Check sheet for the modelled part. Datum: model origin and axes. Units: mm. A direction names the side the tool comes from. Round coordinates to 2 decimals unless told otherwise and drop trailing zeros. Loops run counter-clockwise (first coordinate to the right, second up) from the corner with the lowest first, then second, coordinate; pieces in that order, holes last. Notation, with made-up numbers: (49, -22.75) - (59, -22.75) arc R20 cw to (59, -8.75) - close; hole circle Ø6 at (18.5, -16). An arc over 180 degrees is marked (long way). Answer in a Markdown table with one row per item. Add a question column.
(1) Cross-section at C-C on z = 12. Count the separate pieces of the cut face and the enclosed holes in it, then the cut area to 3 significant figures.
(2) Gauge pin test, flat ends, axial feed: pin 1 (12.5 mm diameter, centred on x = 16.5, z = 8.5, fed in from +Y); pin 2 (12 mm diameter, centred on x = 15.5, y = -6, fed in from -Z) (3 decimals); pin 3 (8 mm diameter, centred on y = -11, z = 10.5, fed in from -X); pin 4 (2 mm diameter, centred on x = 33, y = -8, fed in from -Z). Record the tip position at first contact, or that the pin passes through.
(3) Cross-section at A-A on x = 36. Enter the section's corners in (y, z).
(4) Cross-section at B-B on z = 30. Enter the section's corners in (x, y) (3 decimals).
(5) Mould release check, pull along X, two halves, no side actions. Record for faces 5 (the flat face through (28, -19, 28.575)), 6 (the flat face through (12.7, -14, 21)), 7 (the flat face through (14, -32.4, 15.8)), 8 (the flat face through (22.2, -33.5, 30.1)): +X half, -X half, draft (parallel to the pull), parting line (faces both ways), or undercut.
(6) Thickness scan on line 1 along Y through (x, z) = (12.5, 20.5); line 2 along Y through (x, z) = (34, 21); line 3 along Y through (x, z) = (17, 10.5). Record the ranges inside material, lowest first.
(7) Access from +Z, -Z, +X, -X, +Y, -Y to the whole of each face (thin tool, end or side, straight path). Record for faces 1 (the flat face through (5.06, -15.83, 7.83)), 2 (the flat face through (19, -22, 9.525)), 3 (the flat face through (12.7, -9, 23)), 4 (the flat face through (25.4, -30, 23)).
(8) Cross-section at D-D on y = -14.5. Enter the section's corners in (x, z) (3 decimals).
from build123d import *

# Parameters (mm, degrees)
F0_W      = 38.1
F0_H      = 38.1
F1_DEPTH  = 38.1
F6_DEPTH  = 38.1
F8_DEPTH  = 38.1
F9_W      = 25.4
F9_H      = 7.62
F10_DEPTH = 38.1
F11_W     = 25.4
F11_H     = 7.62
F12_DEPTH = 38.1


with BuildPart() as f1:
    # F0 (on Front) → F1 (new body)
    with BuildSketch(Plane.XZ):
        with Locations((19.05, 19.05)):
            Rectangle(F0_W, F0_H)
    extrude(amount=F1_DEPTH)

    # F5 (on offset) → F6 (cut)
    with BuildSketch(Plane.YZ.offset(38.1)):
        Polygon((-31.75, 0), (-38.1, 38.1), (-38.1, 0), align=None)
        Polygon((-19.05, 15.875), (-25.4, 0), (-12.7, 0), align=None)
        Polygon((0, 0), (0, 38.1), (-6.35, 0), align=None)
        Polygon((-6.35, 38.1), (-31.75, 38.1), (-26.67, 17.949333), (-21.59, 28.575), (-16.51, 28.575), (-11.43, 17.78), align=None)
    extrude(amount=-F6_DEPTH, mode=Mode.SUBTRACT)

    # F7 (on offset) → F8 (cut)
    with BuildSketch(Plane.XZ.offset(38.1)):
        Polygon((25.4, 38.1), (12.7, 38.1), (19.05, 22.225), align=None)
        Polygon((6.35, 38.1), (0, 38.1), (0, 0), align=None)
        Polygon((11.43, 22.225), (6.35, 0), (31.75, 0), (26.67, 22.225), (21.59, 9.525), (16.51, 9.525), align=None)
        Polygon((38.1, 38.1), (31.75, 38.1), (38.1, 0), align=None)
    extrude(amount=-F8_DEPTH, mode=Mode.SUBTRACT)

    # F9 (on Top) → F10 (cut)
    with BuildSketch(Plane.XY):
        with Locations((12.7, -26.67)):
            Rectangle(F9_W, F9_H)
        with Locations((25.4, -11.43)):
            Rectangle(F9_W, F9_H)
    extrude(amount=-F10_DEPTH, mode=Mode.SUBTRACT)

    # F11 (on offset) → F12 (cut)
    with BuildSketch(Plane.XY.offset(38.1)):
        with Locations((12.7, -26.67)):
            Rectangle(F11_W, F11_H)
        with Locations((25.4, -11.43)):
            Rectangle(F11_W, F11_H)
    extrude(amount=-F12_DEPTH, mode=Mode.SUBTRACT)


solid = f1.part
Answers:
| question | item | result |
|---|---|---|
| 1 | separate pieces | 10 |
| 1 | enclosed holes | 0 |
| 1 | area | 343 mm^2 |
| 2 | pin 1 | stops at y = -3.89 |
| 2 | pin 2 | stops at z = 9.525 |
| 2 | pin 3 | stops at x = 1.08 |
| 2 | pin 4 | stops at z = 0 |
| 3 | outline | (-33.85, 12.6) - (-31.75, 0) - (-25.4, 0) - (-20.36, 12.6) - close; (-17.74, 12.6) - (-15.24, 6.35) - (-15.24, 12.6) - close; (-7.62, 0) - (-6.35, 0) - (-4.25, 12.6) - (-7.62, 12.6) - close |
| 4 | outline | (5, -36.75) - (15.94, -36.75) - (15.94, -30.48) - (5, -30.48) - close; (5, -8.375) - (12.7, -8.375) - (12.7, -7.62) - (15.94, -7.62) - (15.94, -1.35) - (5, -1.35) - close; (22.16, -36.75) - (33.1, -36.75) - (33.1, -29.708) - (25.4, -29.708) - (25.4, -30.48) - (22.16, -30.48) - close; (22.16, -7.62) - (33.1, -7.62) - (33.1, -1.35) - (22.16, -1.35) - close |
| 5 | face 5 | draft |
| 5 | face 6 | +X half |
| 5 | face 7 | undercut |
| 5 | face 8 | undercut |
| 6 | line 1 | y = -35.17 to -30.48, -22.86 to -12.71, -10.75 to -2.93 |
| 6 | line 2 | y = -35.25 to -27.44, -25.21 to -15.24, -7.62 to -2.85 |
| 6 | line 3 | y = -33.5 to -30.48, -22.86 to -21.2, -16.9 to -15.24, -7.62 to -4.6 |
| 7 | face 1 | -Z, +X, -X |
| 7 | face 2 | -Z, +Y, -Y |
| 7 | face 3 | +Z, -Z, +X |
| 7 | face 4 | +Z, -Z, -X |
| 8 | outline | (0.75, 4.5) - (7.379, 4.5) - (11.43, 22.225) - (12.7, 19.05) - (12.7, 24.304) - (4.051, 24.304) - close |
